```python
from build123d import *

# Parameters (mm, degrees)
ESQUISSE1_R             = 11
ESQUISSE1_R_2           = 1.6
BOSS_EXTRU_1_DEPTH      = 2.5
ESQUISSE2_W             = 50
ESQUISSE2_H             = 2.5
BOSS_EXTRU_2_DEPTH      = 49
ENL_V_MAT_EXTRU_1_DEPTH = 94.737929077
CONG_1_R                = 3
CONG_2_R                = 2
BOSS_EXTRU_3_DEPTH      = 2


with BuildPart() as part:
    # Esquisse1 → Boss.-Extru.1 (new body)
    with BuildSketch(Plane(origin=(0, 0, 0), x_dir=(-1, 0, 0), z_dir=(0, 0, -1))):
        with BuildLine():
            Line((-11.5004012, -0.849780391), (-11.5004012, 49.150219609))
            ThreePointArc((-11.5004012, 49.150219609), (-11.793294419, 49.85732639), (-12.5004012, 50.150219609))
            Line((-12.5004012, 50.150219609), (-60.5004012, 50.150219609))
            ThreePointArc((-60.5004012, 50.150219609), (-61.207507981, 49.85732639), (-61.5004012, 49.150219609))
            Line((-61.5004012, 49.150219609), (-61.5004012, -0.849780391))
            Line((-61.5004012, -0.849780391), (-11.5004012, -0.849780391))
        make_face()
        with Locations((-36.5004012, 30.150219609)):
            Circle(ESQUISSE1_R, mode=Mode.SUBTRACT)
        with Locations((-52.0004012, 14.650219609)):
            Circle(ESQUISSE1_R_2, mode=Mode.SUBTRACT)
        with Locations((-52.000444233, 45.650219609)):
            Circle(ESQUISSE1_R_2, mode=Mode.SUBTRACT)
        with Locations((-21.0004012, 14.650219609)):
            Circle(ESQUISSE1_R_2, mode=Mode.SUBTRACT)
        with Locations((-21.0004012, 45.650219609)):
            Circle(ESQUISSE1_R_2, mode=Mode.SUBTRACT)
    extrude(amount=-BOSS_EXTRU_1_DEPTH)

    # Esquisse2 → Boss.-Extru.2 (add)
    with BuildSketch(Plane.XY.offset(2.5)):
        with Locations((36.5004012, 0.400219609)):
            Rectangle(ESQUISSE2_W, ESQUISSE2_H)
    extrude(amount=BOSS_EXTRU_2_DEPTH)

    # Esquisse5 → Enlèv. mat.-Extru.1 (cut, through all)
    with BuildSketch(Plane(origin=(0, 1.650219609, 0), x_dir=(1, 0, 0), z_dir=(0, 1, 0))):
        with BuildLine():
            Line((23.6004012, -11.5), (23.6004012, -41.3))
            ThreePointArc((23.6004012, -41.3), (21.5004012, -43.4), (19.4004012, -41.3))
            Line((19.4004012, -41.3), (19.4004012, -11.5))
            ThreePointArc((19.4004012, -11.5), (21.5004012, -9.4), (23.6004012, -11.5))
        make_face()
        with BuildLine():
            Line((49.4004012, -11.5), (49.4004012, -41.3))
            ThreePointArc((49.4004012, -41.3), (51.5004012, -43.4), (53.6004012, -41.3))
            Line((53.6004012, -41.3), (53.6004012, -11.5))
            ThreePointArc((53.6004012, -11.5), (51.5004012, -9.4), (49.4004012, -11.5))
        make_face()
    extrude(amount=-ENL_V_MAT_EXTRU_1_DEPTH, mode=Mode.SUBTRACT)

    # Congé1
    cong_1_edges = [part.edges().sort_by_distance(p)[0] for p in [
        (36.5004012, -0.849780391, 0),
    ]]
    fillet(cong_1_edges, radius=CONG_1_R)

    # Congé2
    cong_2_edges = [part.edges().sort_by_distance(p)[0] for p in [
        (36.5004012, 1.650219609, 2.5),
    ]]
    fillet(cong_2_edges, radius=CONG_2_R)

    # Esquisse4 → Boss.-Extru.3 (add)
    with BuildSketch(Plane.ZY.offset(-11.5004012)):
        Polygon((1.986701053, 6.637130702), (6.116686164, 1.109304476), (13.296506434, 1.109304476), (1.986701053, 21.949844729), align=None)
    boss_extru_3 = extrude(amount=-BOSS_EXTRU_3_DEPTH)

    # Symétrie1: Boss.-Extru.3 across plane
    add(boss_extru_3.mirror(Plane.ZY.offset(-36.5004012)))


solid = part.part
```
Geometry: final body of the model. Coordinates: model frame, mm. A direction names the side the tool comes from. Round coordinates to 2 decimals unless told otherwise and drop trailing zeros. Order: outer loops, then holes, each group sorted by start corner. A loop starts at its lowest first (then second) coordinate and runs counter-clockwise, first axis right, second up. Notation, with made-up numbers: (-24.5, 58) - (-2.5, 58) arc R6 ccw to (-2.5, 66) - close; hole circle Ø11 at (53, 35). An arc over 180 degrees is marked (long way). Use CSV: the item, a comma, the result in double quotes. Start each with the question number.
Q1. Section query C-C (x = 46.5). Return loops of the section in (y, z).
Q2. Section query B-B (x = 51.5). Return loops of the section in (y, z).
Q3. Mould query, pull axis Z, two halves, no side actions, for faces 1 (the face through (13.5, 9, 7)), 2 (the face through (36, 0, 51.5)), 3 (the face through (51.5, 0.4, 9.4)). Classes: +Z half, -Z half, draft (parallel to the pull), parting line (faces both ways), or undercut.
Q4. Section query A-A (z = 15). Return loops of the section in (x, y), and give its area (3 significant figures).
Q5. Material intervals for line 1 along Y through (x, z) = (37.5, 24); line 2 along Z through (x, y) = (52.5, 8.5); line 3 along Y through (x, z) = (32.5, 3.5), sorted ascending. Write a range as from..to.
Q6. Section query D-D (x = 57). Return loops of the section in (y, z), and give its area (3 significant figures).
Q7. First-contact query: pin 1 (3.5 mm diameter, centred on x = 52, y = 45.65, fed in from +Z); pin 2 (2 mm diameter, centred on x = 46, z = 19, fed in from +Y). Flat tips, straight axial feed; report the tip coordinate or a pass-through.
Q8. Access query for faces 4 (the face through (61.5, 9, 8)), 5 (the face through (49.4, 0, 26)). Directions: +Z, -Z, +X, -X, +Y, -Y. A direction counts if a zero-diameter tool reaches every point of the face in a straight line with its end or side. Return the directions, or none.
Result set:
1,outline,"(-0.85, 3) arc R3 ccw to (2.15, 0) - (25.57, 0) - (25.57, 2.5) - (3.65, 2.5) arc R2 cw to (1.65, 4.5) - (1.65, 51.5) - (-0.85, 51.5) - close; (34.73, 0) - (50.15, 0) - (50.15, 2.5) - (34.73, 2.5) - close"
2,outline,"(-0.85, 3) arc R3 ccw to (2.15, 0) - (13.13, 0) - (13.13, 2.5) - (3.65, 2.5) arc R2 cw to (1.65, 4.5) - (1.65, 9.4) - (-0.85, 9.4) - close; (-0.85, 43.4) - (1.65, 43.4) - (1.65, 51.5) - (-0.85, 51.5) - close; (16.17, 0) - (44.13, 0) - (44.13, 2.5) - (16.17, 2.5) - close; (47.17, 0) - (50.15, 0) - (50.15, 2.5) - (47.17, 2.5) - close"
3,face 1,"draft"
3,face 2,"+Z half"
3,face 3,"undercut"
4,outline,"(11.5, -0.85) - (19.4, -0.85) - (19.4, 1.65) - (11.5, 1.65) - close; (23.6, -0.85) - (49.4, -0.85) - (49.4, 1.65) - (23.6, 1.65) - close; (53.6, -0.85) - (61.5, -0.85) - (61.5, 1.65) - (53.6, 1.65) - close"
4,area,"104 mm2"
5,line 1,"y = -0.85..1.65"
5,line 2,"z = 0..2.5"
5,line 3,"y = -0.85..1.92"
6,outline,"(-0.85, 3) arc R3 ccw to (2.15, 0) - (50.15, 0) - (50.15, 2.5) - (3.65, 2.5) arc R2 cw to (1.65, 4.5) - (1.65, 51.5) - (-0.85, 51.5) - close"
6,area,"249 mm2"
7,pin 1,"stops at z = 2.5"
7,pin 2,"stops at y = 1.65"
8,face 4,"+Z, -Z, +X, +Y, -Y"
8,face 5,"+Y, -Y"
